Check sheet for the modelled part. Datum: model origin and axes. Units: mm. Face numbers are marked on the shaded views. A direction names the side the tool comes from. Give positions to 0.01 mm unless a question says otherwise; leave off trailing zeros. Write each loop counter-clockwise with the first axis right and the second up, starting at its lowest first coordinate (ties: lowest second). Pieces come first, ordered by that corner, then holes. Notation, with made-up numbers: (54, 47) -> (60, 47) arc R5 ccw to (60, 54) -> close; hole circle Ø5 at (51, 15). An arc over 180 degrees is marked (long way). Use a Markdown table: item, result. Add a question column.
1. Cross-section at C-C (y = -13). Enter the section's corners in (x, z), then the cut area to 3 significant figures.
2. Scan lines: probe 1 along Y at (x, z) = (-20, -5); probe 2 along Z at (x, y) = (-41, -2.5); probe 3 along X at (y, z) = (-1, -2). Record each from-to range of solid material in increasing order. Write a range as [from, to].
3. Set-up check for the marked faces 1 and 2: record each of +Z, -Z, +X, -X, +Y, -Y from which the full face is reachable in a straight line by a thin tool's end or side.
4. Cross-section at B-B (z = -2). Enter the section's corners in (x, y), then the cut area to 3 significant figures.
5. Release check for a two-part mould opening along Y. For the marked faces 3, 4 and 5 record: released by +Y, released by -Y, zero draft, split by the parting line, or undercut.
6. Cross-section at A-A (x = -31). Enter the section's corners in (y, z), then the cut area to 3 significant figures.
7. Gauge pin test, flat ends, axial feed: P1, Ø1, axis at x = 84, y = -44, coming from the -Z side; P2, Ø4, axis at y = 28.5, z = 2.5, coming from the +X side; P3, Ø1.5, axis at x = 8.5, z = -10, coming from the -Y side. Record the tip position at first contact, or that the pin passes through.
from build123d import *

# Parameters (mm, degrees)
F0_W     = 190
F0_H     = 90
F1_DEPTH = 30
F2_T     = -2
F4_DEPTH = 20
F3_W     = 0.1180022955
F3_H     = 85.8825759888
F3_W_2   = 1.8819977045
F5_DEPTH = 20
F6_W     = 7
F6_H     = 9
F7_DEPTH = 4
F8_W     = 7
F8_H     = 9
F9_DEPTH = 4


with BuildPart() as f1:
    # F0 (on Top) → F1 (new body)
    with BuildSketch(Plane.XY):
        Rectangle(F0_W, F0_H)
    extrude(amount=F1_DEPTH)

    # F2
    f2_openings = [f1.faces().sort_by_distance(p)[0] for p in [
        (95, 0, 15),
    ]]
    offset(amount=F2_T, openings=f2_openings)

    # F3 (on Top) → F4 (join)
    with BuildSketch(Plane.XY):
        Polygon((95.0710946321, 42.9269237816), (95.0710946321, 44.9269237816), (-94.9289053679, 44.9269237816), (-94.9289053679, 42.9269237816), (-93.0469076633, 42.9269237816), (93.0710946321, 42.9269237816), align=None)
    extrude(amount=-F4_DEPTH)

    # F3 (on Top) → F5 (join)
    with BuildSketch(Plane.XY):
        Polygon((95.0710946321, 42.9269237816), (95.0710946321, 44.9269237816), (-94.9289053679, 44.9269237816), (-94.9289053679, 42.9269237816), (-93.0469076633, 42.9269237816), (93.0710946321, 42.9269237816), align=None)
        Polygon((95.0710946321, -42.9556522071), (95.0710946321, 42.9269237816), (93.0710946321, 42.9269237816), (93.0710946321, -42.9556522071), (94.9564541443, -42.9556522071), align=None)
        with Locations((-94.9879065156, -0.0143642128)):
            Rectangle(F3_W, F3_H)
        with Locations((-93.9879065156, -0.0143642128)):
            Rectangle(F3_W_2, F3_H)
        Polygon((-93.0469076633, -42.9556522071), (-94.9289053679, -42.9556522071), (-95.0469076633, -42.9556522071), (-95.0469076633, -44.9556522071), (94.9533249005, -44.9556522071), (94.9564541443, -42.9556522071), (93.0710946321, -42.9556522071), align=None)
    extrude(amount=-F5_DEPTH)

    # F6 (on face) → F7 (cut)
    with BuildSketch(Plane(origin=(0, 44.9269237816, 0), x_dir=(-1, 0, 0), z_dir=(0, 1, 0))):
        with Locations((13.4289053679, -15.5)):
            Rectangle(F6_W, F6_H)
        with Locations((-0.5710946321, -15.5)):
            Rectangle(F6_W, F6_H)
        with Locations((-14.5710946321, -15.5)):
            Rectangle(F6_W, F6_H)
        with Locations((-28.5710946321, -15.5)):
            Rectangle(F6_W, F6_H)
        with Locations((-42.5710946321, -15.5)):
            Rectangle(F6_W, F6_H)
        with Locations((-56.5710946321, -15.5)):
            Rectangle(F6_W, F6_H)
        with Locations((-70.5710946321, -15.5)):
            Rectangle(F6_W, F6_H)
        with Locations((-84.5710946321, -15.5)):
            Rectangle(F6_W, F6_H)
    extrude(amount=-F7_DEPTH, mode=Mode.SUBTRACT)

    # F8 (on face) → F9 (cut)
    with BuildSketch(Plane.XZ.offset(44.9556522071)):
        with Locations((84.4533249005, -15.5)):
            Rectangle(F8_W, F8_H)
        with Locations((70.4533249005, -15.5)):
            Rectangle(F8_W, F8_H)
        with Locations((56.4533249005, -15.5)):
            Rectangle(F8_W, F8_H)
        with Locations((42.4533249005, -15.5)):
            Rectangle(F8_W, F8_H)
        with Locations((28.4533249005, -15.5)):
            Rectangle(F8_W, F8_H)
        with Locations((14.4533249005, -15.5)):
            Rectangle(F8_W, F8_H)
        with Locations((0.4533249005, -15.5)):
            Rectangle(F8_W, F8_H)
        with Locations((-13.5466750995, -15.5)):
            Rectangle(F8_W, F8_H)
    extrude(amount=-F9_DEPTH, mode=Mode.SUBTRACT)


solid = f1.part
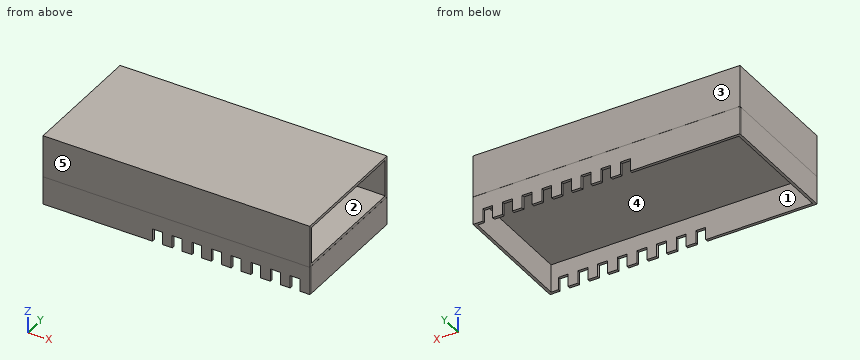
Worked answers:
| question | item | result |
|---|---|---|
| 1 | outline | (-95.05, -20) -> (-93.05, -20) -> (-93.05, 0) -> (93.07, 0) -> (93.07, -20) -> (95.07, -20) -> (95.07, 0) -> (95, 0) -> (95, 2) -> (-93, 2) -> (-93, 28) -> (95, 28) -> (95, 30) -> (-95, 30) -> (-95, 0) -> (-95.05, 0) -> close |
| 1 | area | 892 mm² |
| 2 | probe 1 | y = [-44.96, -42.96], [42.93, 44.93] |
| 2 | probe 2 | z = [0, 2], [28, 30] |
| 2 | probe 3 | x = [-95.05, -93.05], [93.07, 95.07] |
| 3 | face 1 | -Z |
| 3 | face 2 | +X |
| 4 | outline | (-95.05, -44.96) -> (94.95, -44.96) -> (94.96, -42.96) -> (95.07, -42.96) -> (95.07, 44.93) -> (-94.93, 44.93) -> (-94.93, 42.93) -> (-95.05, 42.93) -> close; hole (-93.05, -42.96) -> (93.07, -42.96) -> (93.07, 42.93) -> (-93.05, 42.93) -> close |
| 4 | area | 1,100 mm² |
| 5 | face 3 | released by +Y |
| 5 | face 4 | undercut |
| 5 | face 5 | released by -Y |
| 6 | outline | (-45, 0) -> (-44.96, 0) -> (-44.96, -20) -> (-42.96, -20) -> (-42.96, 0) -> (42.93, 0) -> (42.93, -20) -> (44.93, -20) -> (44.93, 0) -> (45, 0) -> (45, 30) -> (-45, 30) -> close; hole (-43, 2) -> (43, 2) -> (43, 28) -> (-43, 28) -> close |
| 6 | area | 544 mm² |
| 7 | P1 | stops at z = -11 |
| 7 | P2 | stops at x = 95 |
| 7 | P3 | stops at y = -44.96 |
